Verification items for the finished model (mm, model axes). A direction names the side the tool comes from. Coordinates: 2 decimals unless noted, no trailing zeros. Order: outer loops, then holes, each group sorted by start corner. A loop starts at its lowest first (then second) coordinate and runs counter-clockwise, first axis right, second up. Notation, with made-up numbers: M 75,-31.5 L 95,-31.5 A23 cw 95,-18.5 Z; hole C 10,35 d3. An arc over 180 degrees is marked long. Answer as a JSON object with one key per item and string values. Group by question number.
(1) Mould release check, pull along Y, two halves, no side actions. Record for faces 1 (the face through (-25.4, 0, -1)), 2 (the face through (-57.15, 22.5, -34.7)), 3 (the face through (0.8, -5.506, -50.196)): released by +Y, released by -Y, zero draft, split by the parting line, or undercut.
(2) Gauge pin test, flat ends, axial feed: pin 1 Ø2 at (x, z) = (-19, -42) entering from +Y; pin 2 Ø10 at (y, z) = (6, -10.5) entering from -X; pin 3 Ø4 at (x, z) = (-44, -39.5) entering from +Y; pin 4 Ø0.7 at (x, z) = (6.5, -4.5) entering from -Y. Record the tip position at first contact, or that the pin passes through.
(3) Cross-section at A-A (z = -37.5). Enter the section's corners in (x, y) (3 decimals).
(4) Cross-section at C-C (x = 41). Enter the section's corners in (y, z).
(5) Cross-section at B-B (y = 2). Enter the section's corners in (x, z).
(6) Material ranges on line 1 (X direction, y = -19.05, z = -9) (3 decimals); line 2 (Y direction, x = -20, z = -25); line 3 (Z direction, x = -9, y = 13), recorded low to high.
(7) Cross-section at D-D (x = 14). Enter the section's corners in (y, z).
(8) Access from +Z, -Z, +X, -X, +Y, -Y to the whole of each face (thin tool, end or side, straight path). Record for faces 4 (the face through (57.15, 22.5, -34.7)), 5 (the face through (25.4, 0, -1)).
from build123d import *

# Parameters (mm, degrees)
F0_R     = 25.4
F1_DEPTH = 57.15
F3_DEPTH = 25.4
F5_DEPTH = 114.3
F7_DEPTH = 76.2


with BuildPart() as f1:
    # F0 (on Right) → F1 (new body, symmetric)
    with BuildSketch(Plane.YZ):
        with Locations((0, -25.4)):
            Circle(F0_R)
    extrude(amount=F1_DEPTH, both=True)

    # F2 (on Top) → F3 (cut)
    with BuildSketch(Plane.XY):
        Polygon((-25.4, 12.7), (-25.4, 0), (-25.4, -12.7), (25.4, -12.7), (25.4, 0), (25.4, 12.7), align=None)
    extrude(amount=-F3_DEPTH, mode=Mode.SUBTRACT)

    # F4 (on face) → F5 (cut)
    with BuildSketch(Plane.YZ.offset(57.15)):
        with BuildLine():
            ThreePointArc((24.13, -25.4), (17.06248663, -8.33751337), (0, -1.27))
            ThreePointArc((0, -1.27), (-17.06248663, -42.46248663), (24.13, -25.4))
        make_face()
    extrude(amount=-F5_DEPTH, mode=Mode.SUBTRACT)

    # F6 (on Top) → F7 (cut)
    with BuildSketch(Plane.XY):
        with BuildLine():
            ThreePointArc((-42.545, -19.05), (-43.4749359697, -16.8049359697), (-45.72, -15.875))
            ThreePointArc((-45.72, -15.875), (-47.9650640303, -21.2950640303), (-42.545, -19.05))
        make_face()
        with BuildLine():
            ThreePointArc((48.895, -19.05), (47.9650640303, -16.8049359697), (45.72, -15.875))
            ThreePointArc((45.72, -15.875), (43.4749359697, -21.2950640303), (48.895, -19.05))
        make_face()
    extrude(amount=-F7_DEPTH, mode=Mode.SUBTRACT)


solid = f1.part
Taken from the geometry:
{
 "1": {"face 1": "undercut", "face 2": "zero draft", "face 3": "split by the parting line"},
 "2": {"pin 1": "stops at y = 20.04", "pin 2": "passes through", "pin 3": "stops at y = 22.33", "pin 4": "stops at y = -14.93"},
 "3": {"outline": "M -57.15,-22.333 L 57.15,-22.333 L 57.15,-20.877 L 48.317,-20.877 A3.175 cw 43.123,-20.877 L -43.123,-20.877 A3.175 cw -48.317,-20.877 L -57.15,-20.877 Z; M -57.15,20.877 L 57.15,20.877 L 57.15,22.333 L -57.15,22.333 Z"},
 "4": {"outline": "C 0,-25.4 d50.8; hole C 0,-25.4 d48.26"},
 "5": {"outline": "M -57.15,-50.72 L 57.15,-50.72 L 57.15,-49.45 L -57.15,-49.45 Z; M -57.15,-1.35 L -25.4,-1.35 L -25.4,-0.08 L -57.15,-0.08 Z; M 25.4,-1.35 L 57.15,-1.35 L 57.15,-0.08 L 25.4,-0.08 Z"},
 "6": {"line 1": "x = -57.15 to -48.895, -42.545 to 42.545, 48.895 to 57.15", "line 2": "y = -25.4 to -24.13, 24.13 to 25.4", "line 3": "z = -47.22 to -45.73, -5.07 to -3.58"},
 "7": {"outline": "M -12.7,-4.88 L -12.7,-3.4 A25.4 ccw long 12.7,-3.4 L 12.7,-4.88 A24.13 cw long Z"},
 "8": {"face 4": "+Z, -Z, +X, +Y, -Y", "face 5": "+Z"}
}
